Geometry: final body of the model. Coordinates: model frame, mm. A direction names the side the tool comes from. Round coordinates to 2 decimals unless told otherwise and drop trailing zeros. Order: outer loops, then holes, each group sorted by start corner. A loop starts at its lowest first (then second) coordinate and runs counter-clockwise, first axis right, second up. Notation, with made-up numbers: (-0.75, -16.75) - (42.25, -16.75) arc R6 ccw to (42.25, -9.75) - close; hole circle Ø3 at (40.5, -15.5). An arc over 180 degrees is marked (long way). Put each result on its own line as item: value. Start each with the question number.
(1) Pin query (flat end, axial travel): P1, Ø12, axis at x = -25.5, y = 21, coming from the -Z side (3 decimals); P2, Ø10, axis at x = 15, y = 36.5, coming from the +Z side (3 decimals); P3, Ø8, axis at x = 1, z = 15.5, coming from the -Y side; P4, Ø1.5, axis at y = 42, z = -5.5, coming from the -X side. Return the tip coordinate at first contact, or that it passes through.
(2) Pull-direction query (Z, two-part tool) for faces 1 (the face through (-12, 6, -2)), 2 (the face through (-48, 3, 49.275)), 3 (the face through (-50.6, 3.04, -39.59)); classes: released by +Z, released by -Z, zero draft, split by the parting line, or undercut.
(3) Access query for faces 4 (the face through (40, 3, 40)), 5 (the face through (26, 26, -2)), 6 (the face through (43, 6, 1)). Directions: +Z, -Z, +X, -X, +Y, -Y. A direction counts if a zero-diameter tool reaches every point of the face in a straight line with its end or side. Return the directions, or none.
(4) Section A-A (x = -47.5). Output: boundary loops of the cut face in (y, z) (3 decimals), and give its area (3 significant figures).
(5) Section B-B (z = -20.5). Output: boundary loops of the cut face in (x, y), and give its area (3 significant figures).
(6) Material intervals for L1, parallel to Z at x = 47.5, y = 2.4 (3 decimals); L2, parallel to X at y = 3, z = 37; L3, parallel to X at y = 31, z = 24.5, sorted ascending. Write a range as [from, to].
(7) Section C-C (x = 0). Output: boundary loops of the cut face in (y, z) (3 decimals), and give its area (3 significant figures).
(8) Section D-D (y = 12.5). Output: boundary loops of the cut face in (x, z) (3 decimals).
from build123d import *

# Parameters (mm, degrees)
SKETCH1_W           = 110
SKETCH1_H           = 62.55
BOSS_EXTRUDE1_DEPTH = 6
CUT_EXTRUDE1_REACH  = 65.554
SKETCH2_R           = 9.5
SKETCH4_W           = 15
SKETCH4_H           = 6
BOSS_EXTRUDE2_DEPTH = 18
SKETCH5_R           = 3.175
CUT_EXTRUDE3_DEPTH  = 18
SKETCH6_W           = 5
SKETCH6_H           = 62.55
BOSS_EXTRUDE3_DEPTH = 40
SKETCH7_W           = 62.55
SKETCH7_H           = 5
BOSS_EXTRUDE4_DEPTH = 62
BOSS_EXTRUDE5_REACH = 88.476
SKETCH8_W           = 52
SKETCH8_H           = 5


with BuildPart() as part:
    # Sketch1 → Boss-Extrude1 (new body)
    with BuildSketch(Plane(origin=(0, 0, 0), x_dir=(1, 0, 0), z_dir=(0, 1, 0))):
        Rectangle(SKETCH1_W, SKETCH1_H)
    extrude(amount=BOSS_EXTRUDE1_DEPTH)

    # Sketch2 → Cut-Extrude1 (cut, up to next)
    with BuildSketch(Plane(origin=(0, 6, 0), x_dir=(1, 0, 0), z_dir=(0, 1, 0)), mode=Mode.PRIVATE) as cut_extrude1_sk1:
        with Locations(Location((0, 2.725, 0), (0, 0, 270))):
            Circle(SKETCH2_R)
    cut_extrude1_tool1 = extrude(cut_extrude1_sk1.sketch, amount=-CUT_EXTRUDE1_REACH, mode=Mode.PRIVATE) & part.part
    add(cut_extrude1_tool1.solids().sort_by_distance((0, 6, -2.725))[0], mode=Mode.SUBTRACT)

    # Sketch4 → Boss-Extrude2 (add)
    with BuildSketch(Plane.XY.offset(31.275)):
        with Locations((-47.5, 3)):
            Rectangle(SKETCH4_W, SKETCH4_H)
        with Locations((47.5, 3)):
            Rectangle(SKETCH4_W, SKETCH4_H)
    boss_extrude2 = extrude(amount=BOSS_EXTRUDE2_DEPTH)

    # Sketch5 → Cut-Extrude3 (cut)
    with BuildSketch(Plane(origin=(0, 6, 0), x_dir=(1, 0, 0), z_dir=(0, 1, 0))):
        with Locations(Location((-47.5, -40.275, 0), (0, 0, 270))):
            Circle(SKETCH5_R)
        with Locations(Location((47.5, -40.275, 0), (0, 0, 90))):
            Circle(SKETCH5_R)
    cut_extrude3 = extrude(amount=-CUT_EXTRUDE3_DEPTH, mode=Mode.SUBTRACT)

    # Mirror1: Boss-Extrude2, Cut-Extrude3 across plane
    add(boss_extrude2.mirror(Plane.XY))
    add(cut_extrude3.mirror(Plane.XY), mode=Mode.SUBTRACT)

    # Sketch6 → Boss-Extrude3 (add)
    with BuildSketch(Plane(origin=(0, 6, 0), x_dir=(1, 0, 0), z_dir=(0, 1, 0))):
        with Locations((28.5, 0)):
            Rectangle(SKETCH6_W, SKETCH6_H)
        with Locations((-28.5, 0)):
            Rectangle(SKETCH6_W, SKETCH6_H)
    extrude(amount=BOSS_EXTRUDE3_DEPTH)

    # Sketch7 → Boss-Extrude4 (add)
    with BuildSketch(Plane(origin=(31, 0, 0), x_dir=(0, 0, -1), z_dir=(1, 0, 0))):
        with Locations((0, 48.5)):
            Rectangle(SKETCH7_W, SKETCH7_H)
    extrude(amount=-BOSS_EXTRUDE4_DEPTH)

    # Sketch8 → Boss-Extrude5 (add, up to next)
    with BuildSketch(Plane(origin=(0, 6, 0), x_dir=(1, 0, 0), z_dir=(0, 1, 0)), mode=Mode.PRIVATE) as boss_extrude5_sk1:
        with Locations((0, -28.775)):
            Rectangle(SKETCH8_W, SKETCH8_H)
    boss_extrude5_tool1 = extrude(boss_extrude5_sk1.sketch, amount=BOSS_EXTRUDE5_REACH, mode=Mode.PRIVATE) - part.part
    add(boss_extrude5_tool1.solids().sort_by_distance((0, 6, 28.775))[0])


solid = part.part
Checks:
1. P1: stops at z = -31.275
1. P2: stops at z = 31.275
1. P3: stops at y = 0
1. P4: stops at x = -31
2. face 1: zero draft
2. face 2: released by +Z
2. face 3: undercut
3. face 4: +Z, +Y, -Y
3. face 5: -Z
3. face 6: +Z, -Z, +X, +Y
4. outline: (0, -49.275) - (6, -49.275) - (6, -43.45) - (0, -43.45) - close; (0, -37.1) - (6, -37.1) - (6, 37.1) - (0, 37.1) - close; (0, 43.45) - (6, 43.45) - (6, 49.275) - (0, 49.275) - close
4. area: 515 mm²
5. outline: (-55, 0) - (55, 0) - (55, 6) - (31, 6) - (31, 51) - (-31, 51) - (-31, 6) - (-55, 6) - close; hole (-26, 6) - (26, 6) - (26, 46) - (-26, 46) - close
5. area: 1,370 mm²
6. L1: z = [-49.275, -43.45], [-37.1, 37.1], [43.45, 49.275]
6. L2: x = [-55, -40], [40, 55]
6. L3: x = [-31, -26], [26, 31]
7. outline: (0, -31.275) - (6, -31.275) - (6, -12.225) - (0, -12.225) - close; (0, 6.775) - (6, 6.775) - (6, 26.275) - (46, 26.275) - (46, -31.275) - (51, -31.275) - (51, 31.275) - (0, 31.275) - close
7. area: 774 mm²
8. outline: (-31, -31.275) - (-26, -31.275) - (-26, 26.275) - (26, 26.275) - (26, -31.275) - (31, -31.275) - (31, 31.275) - (-31, 31.275) - close
